```python
from build123d import *

# Parameters (mm, degrees)
SKETCH3_W           = 25.4
SKETCH3_H           = 25.4
SKETCH3_W_2         = 19.05
SKETCH3_H_2         = 19.05
BOSS_EXTRUDE2_DEPTH = 322.58
CUT_EXTRUDE2_DEPTH  = 299.72
CUT_EXTRUDE3_DEPTH  = 25.4


with BuildPart() as part:
    # Sketch3 → Boss-Extrude2 (new body)
    with BuildSketch(Plane.XY):
        with Locations((-2.765581944, -1.754080231)):
            Rectangle(SKETCH3_W, SKETCH3_H)
        with Locations((-2.765581944, -1.754080231)):
            Rectangle(SKETCH3_W_2, SKETCH3_H_2, mode=Mode.SUBTRACT)
    extrude(amount=BOSS_EXTRUDE2_DEPTH)

    # Sketch4 → Cut-Extrude2 (cut)
    with BuildSketch(Plane.ZY.offset(15.465581944)):
        Polygon((322.58, 10.945919769), (297.18, -14.454080231), (322.58, -14.454080231), align=None)
    extrude(amount=-CUT_EXTRUDE2_DEPTH, mode=Mode.SUBTRACT)

    # Sketch5 → Cut-Extrude3 (cut)
    with BuildSketch(Plane.ZY.offset(15.465581944)):
        Polygon((0, -14.454080231), (25.4, 10.945919769), (0, 10.945919769), align=None)
    extrude(amount=-CUT_EXTRUDE3_DEPTH, mode=Mode.SUBTRACT)


solid = part.part
```
Input: part model. Units: mm. Frame: model coordinates. A direction names the side the tool comes from. Round coordinates to 2 decimals unless told otherwise and drop trailing zeros. Loops run counter-clockwise (first coordinate to the right, second up) from the corner with the lowest first, then second, coordinate; pieces in that order, holes last. Notation, with made-up numbers: (29.5, -15) -> (45.5, -15) arc R19 cw to (45.5, 0) -> close; hole circle Ø11 at (22.5, 15.25). An arc over 180 degrees is marked (long way). Use one line per item in the form item = value. Start each with the question number.
Item 1: Section query A-A on x = -2. Return the cut outline in (y, z) (3 decimals), then the cut area to 3 significant figures.
Item 2: Material intervals for L1, parallel to X at y = -4, z = 126.5; L2, parallel to Y at x = 4.25, z = 289; L3, parallel to Y at x = 0, z = 22, sorted ascending. Write a range as from..to.
Item 3: Contact query for flat-ended pins moving along their axis: pin 1 Ø3 at (x, y) = (-11, -5) entering from +Z; pin 2 Ø8 at (x, y) = (-10.5, 1) entering from -Z. Output: stop coordinate, or through.
Item 4: Set-up query: faces 1 (the face through (-3, 10.946, 172)), 2 (the face through (-3, -11.279, 150)). Return all of +Z, -Z, +X, -X, +Y, -Y with unobstructed straight access to the full face (end or side cutting, diameter ignored); none if empty.
Item 5: Mould query, pull axis Y, two halves, no side actions, for faces 3 (the face through (-12.291, -2, 159)), 4 (the face through (8.346, -1.932, 12.522)), 5 (the face through (8.346, -1.576, 310.058)). Classes: pulls with the +Y half, pulls with the -Y half, needs draft (parallel to the pull), parting line crosses it, or undercut.
Item 6: Section query C-C on y = 3. Return the cut outline in (x, z), then the cut area to 3 significant figures.
Item 7: Section query B-B on z = 33.5. Return the cut outline in (x, y), then the cut area to 3 significant figures.
Ans:
q1.outline = (-14.454, 0) -> (-11.279, 3.175) -> (-11.279, 300.355) -> (-14.454, 297.18) -> close; (7.771, 22.225) -> (10.946, 25.4) -> (10.946, 322.58) -> (7.771, 319.405) -> close
q1.area = 1,890 mm^2
q2.L1 = -15.47..-12.29, 6.76..9.93
q2.L2 = -14.45..-11.28, 7.77..10.95
q2.L3 = -14.45..-11.28
q3.pin_1 = 307.4
q3.pin_2 = 11.88
q4.face_1 = +Z, -Z, +X, -X, +Y
q4.face_2 = +Z, -Z
q5.face_3 = undercut
q5.face_4 = pulls with the +Y half
q5.face_5 = pulls with the -Y half
q6.outline = (-15.47, 17.45) -> (-12.29, 17.45) -> (-12.29, 314.63) -> (-15.47, 314.63) -> close; (6.76, 17.45) -> (9.93, 17.45) -> (9.93, 314.63) -> (6.76, 314.63) -> close
q6.area = 1,890 mm^2
q7.outline = (-15.47, -14.45) -> (9.93, -14.45) -> (9.93, 10.95) -> (-15.47, 10.95) -> close; hole (-12.29, -11.28) -> (6.76, -11.28) -> (6.76, 7.77) -> (-12.29, 7.77) -> close
q7.area = 282 mm^2
